Part model, mm, in its own coordinate system. Round coordinates to 2 decimals unless told otherwise and drop trailing zeros. Loops run counter-clockwise (first coordinate to the right, second up) from the corner with the lowest first, then second, coordinate; pieces in that order, holes last. Notation, with made-up numbers: (83.5, -14.75) - (103.5, -14.75) arc R20 ccw to (103.5, 18.25) - close; hole circle Ø3 at (73.25, 33.25). An arc over 180 degrees is marked (long way). Write each question's results on one line, items separated by ' | '. Start each with the question number.
(1) Cut at B-B, the plane z = 2.25. Give the number of separate pieces and of enclosed holes in the cut face, then the cut area to 3 significant figures.
(2) Drill centre lines: L1, parallel to X at y = 0, z = 0.65; L2, parallel to Y at x = 0, z = 1; L3, parallel to X at y = -139.7, z = 1.3. Where is each one in solid material? Low to high.
(3) Cut at A-A, the plane x = 0. List the corners of the cut face in (y, z).
(4) Cut at C-C, the plane y = 21.5. List the corners of the cut face in (x, z).
(5) Cut at D-D, the plane x = 222.5. List the corners of the cut face in (y, z).
Autodesk Inventor part; units mm, degrees
ref_plane "YZ Plane" through (0, 0, 0) normal (1, 0, 0) x (0, 1, 0)
ref_plane "XZ Plane" through (0, 0, 0) normal (0, 1, 0) x (-1, 0, 0)
ref_plane "XY Plane" through (0, 0, 0) normal (0, 0, 1) x (1, 0, 0)
sketch "Sketch1" plane through (0, 0, 0) normal (0, 0, 1) x (1, 0, 0)
  arc A0 (-6.574, 24.5345) -> (-4.4107, -25.0141) centre (0, 0) ccw
  line L0 (-4.4107, -25.0141) -> (146.1169, -51.5562)
  line L1 (146.1169, -51.5562) -> (237.6232, -146.3165)
  arc A1 (237.6232, -146.3165) -> (254, -139.7) centre (244.475, -139.7) ccw
  line L2 (-83.3652, 0) -> (314.9884, 0) construction
  line L3 (254, -139.7) -> (254, 0)
  arc A2 (254, 0) -> (237.5413, 89.945) centre (0, 0) ccw
  line L4 (237.5413, 89.945) -> (-6.574, 24.5345)
  dimension "d1" = 9.525
  dimension "d2" = 25.4
  dimension "d3" = 10
  dimension "d4" = 46.001
  dimension "d6" = 254
  dimension "d7" = 139.7
  dimension "d8" = 15
extrude "Plate1" add sketch "Sketch1" along normal blind 3.048
sketch "Sketch2" plane through (0, 0, 3.048) normal (0, 0, 1) x (1, 0, 0)
  point P0 (0, 0)
  point P1 (0, 0)
hole "Hole1" at (0, 0, 3.048) direction (0, 0, -1) diameter 9.525 end through all
sketch "Sketch3" plane through (0, 0, 3.048) normal (0, 0, 1) x (1, 0, 0)
  arc A0 (237.6232, -146.3165) -> (254, -139.7) centre (244.475, -139.7) ccw construction
  point P0 (0, 0)
hole "Hole2" at (244.475, -139.7, 3.048) direction (0, 0, -1) diameter 6.7564 end through all
equation "\"d14\" = Thickness"
equation "\"d0\" = Thickness"
equation "\"BendRadius\" = Thickness"
equation "\"BendReliefWidth\" = Thickness"
equation "\"BendReliefDepth\" = 0.5 * Thickness"
equation "\"CornerReliefSize\" = 4 * Thickness"
equation "\"MinimumRemnant\" = 2 * Thickness"
equation "\"TransitionRadius\" = BendRadius"
equation "\"JacobiRadiusSize\" = BendRadius"
equation "\"GapSize\" = Thickness"
properties part number "PLATE,ARM,DROPBAR" material "Polycarbonate, Clear"
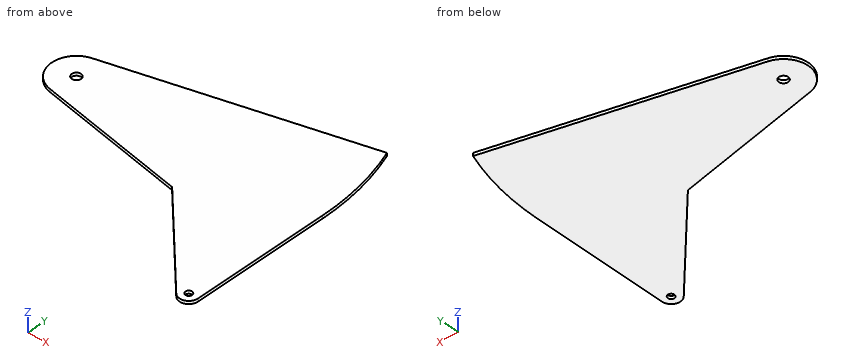
A:
1) separate pieces: 1 | enclosed holes: 2 | area: 32,800 mm2
2) L1: -25.4 to -4.76, 4.76 to 254 | L2: -25.79 to -4.76, 4.76 to 26.3 | L3: 231.23 to 241.1, 247.85 to 254
3) outline: (-25.79, 0) - (-4.76, 0) - (-4.76, 3.05) - (-25.79, 3.05) - close; (4.76, 0) - (26.3, 0) - (26.3, 3.05) - (4.76, 3.05) - close
4) outline: (-13.52, 0) - (253.09, 0) - (253.09, 3.05) - (-13.52, 3.05) - close
5) outline: (-130.66, 0) - (85.91, 0) - (85.91, 3.05) - (-130.66, 3.05) - close
